Here's how the part is built. I have some questions about the finished solid (model axes, mm). A direction names the side the tool comes from. Round coordinates to 2 decimals unless told otherwise and drop trailing zeros. Loops run counter-clockwise (first coordinate to the right, second up) from the corner with the lowest first, then second, coordinate; pieces in that order, holes last. Notation, with made-up numbers: M -20.75,-40 L -0.75,-40 A13 cw -0.75,-27 Z; hole C 21.25,14 d1. An arc over 180 degrees is marked long. Put each result on its own line as item: value. Start each with the question number.
```python
from build123d import *

# Parameters (mm, degrees)
SKETCH_1_W          = 147
SKETCH_1_H          = 50
SKETCH_1_R          = 1.5
EXTRUDE_1_DEPTH     = 2
CUT_EXTRUDE_1_DEPTH = 2
FILLET_2_DEPTH      = 2
FILLET_3_R          = 4
CUT_EXTRUDE_3_DEPTH = 78.661122835
SKETCH_7_R          = 1.75
CUT_EXTRUDE_4_DEPTH = 78.661122835
CUT_EXTRUDE_5_DEPTH = 10
FILLET_4_R          = 1


with BuildPart() as part:
    # 草图1 → 凸台-拉伸1 (new body)
    with BuildSketch(Plane(origin=(0, 0, 0), x_dir=(1, 0, 0), z_dir=(0, 1, 0))):
        Rectangle(SKETCH_1_W, SKETCH_1_H)
        with Locations(Location((18, -18, 0), (0, 0, 270))):
            Circle(SKETCH_1_R, mode=Mode.SUBTRACT)
        with Locations(Location((-18, -18, 0), (0, 0, 270))):
            Circle(SKETCH_1_R, mode=Mode.SUBTRACT)
        with Locations(Location((-18, 18, 0), (0, 0, 270))):
            Circle(SKETCH_1_R, mode=Mode.SUBTRACT)
        with Locations(Location((18, 18, 0), (0, 0, 270))):
            Circle(SKETCH_1_R, mode=Mode.SUBTRACT)
    extrude(amount=EXTRUDE_1_DEPTH)

    # 草图3 → 切除-拉伸1 (cut)
    with BuildSketch(Plane(origin=(0, 2, 0), x_dir=(1, 0, 0), z_dir=(0, 1, 0))):
        with BuildLine():
            Line((-13.345416088, 16.173843213), (0, 2.828427125))
            Line((0, 2.828427125), (13.345416088, 16.173843213))
            ThreePointArc((13.345416088, 16.173843213), (13.868972045, 20.816843629), (18, 23))
            Line((18, 23), (-18, 23))
            ThreePointArc((-18, 23), (-14.464466094, 21.535533906), (-13, 18))
            ThreePointArc((-13, 18), (-13.087112888, 17.070731352), (-13.345416088, 16.173843213))
        make_face()
        with BuildLine():
            Line((16.173843213, 13.345416088), (2.828427125, 0))
            Line((2.828427125, 0), (16.173843213, -13.345416088))
            ThreePointArc((16.173843213, -13.345416088), (20.816843629, -13.868972045), (23, -18))
            Line((23, -18), (23, 18))
            ThreePointArc((23, 18), (20.816843629, 13.868972045), (16.173843213, 13.345416088))
        make_face()
        with BuildLine():
            Line((0, -2.828427125), (-13.345416088, -16.173843213))
            ThreePointArc((-13.345416088, -16.173843213), (-13.087112888, -17.070731352), (-13, -18))
            ThreePointArc((-13, -18), (-14.464466094, -21.535533906), (-18, -23))
            Line((-18, -23), (18, -23))
            ThreePointArc((18, -23), (13.868972045, -20.816843629), (13.345416088, -16.173843213))
            Line((13.345416088, -16.173843213), (0, -2.828427125))
        make_face()
        with BuildLine():
            ThreePointArc((-23, -18), (-20.816843629, -13.868972045), (-16.173843213, -13.345416088))
            Line((-16.173843213, -13.345416088), (-2.828427125, 0))
            Line((-2.828427125, 0), (-16.173843213, 13.345416088))
            ThreePointArc((-16.173843213, 13.345416088), (-20.816843629, 13.868972045), (-23, 18))
            Line((-23, 18), (-23, -18))
        make_face()
    extrude(amount=-CUT_EXTRUDE_1_DEPTH, mode=Mode.SUBTRACT)

    # 圆角2: read off the stored shape, not the designer's step
    # 圆角2 outline → 圆角2 (add)
    with BuildSketch(Plane(origin=(0, 0, 0), x_dir=(1, 0, 0), z_dir=(0, 1, 0))):
        with BuildLine():
            Line((-23, 18), (-23, 9.05572809))
            ThreePointArc((-23, 9.05572809), (-21.666666667, 12.03715206), (-18.555555556, 13.03096005))
            ThreePointArc((-18.555555556, 13.03096005), (-21.726779962, 14.666666667), (-23, 18))
        make_face()
        with BuildLine():
            ThreePointArc((-18.555555556, -13.03096005), (-21.666666667, -12.03715206), (-23, -9.05572809))
            Line((-23, -9.05572809), (-23, -18))
            ThreePointArc((-23, -18), (-21.726779962, -14.666666667), (-18.555555556, -13.03096005))
        make_face()
        with BuildLine():
            ThreePointArc((13.03096005, -18.555555556), (12.03715206, -21.666666667), (9.05572809, -23))
            Line((9.05572809, -23), (18, -23))
            ThreePointArc((18, -23), (14.666666667, -21.726779962), (13.03096005, -18.555555556))
        make_face()
        with BuildLine():
            ThreePointArc((-9.05572809, -23), (-12.03715206, -21.666666667), (-13.03096005, -18.555555556))
            ThreePointArc((-13.03096005, -18.555555556), (-14.666666667, -21.726779962), (-18, -23))
            Line((-18, -23), (-9.05572809, -23))
        make_face()
        with BuildLine():
            ThreePointArc((18.555555556, 13.03096005), (21.666666667, 12.03715206), (23, 9.05572809))
            Line((23, 9.05572809), (23, 18))
            ThreePointArc((23, 18), (21.726779962, 14.666666667), (18.555555556, 13.03096005))
        make_face()
        with BuildLine():
            ThreePointArc((23, -9.05572809), (21.666666667, -12.03715206), (18.555555556, -13.03096005))
            ThreePointArc((18.555555556, -13.03096005), (21.726779962, -14.666666667), (23, -18))
            Line((23, -18), (23, -9.05572809))
        make_face()
        with BuildLine():
            ThreePointArc((-13.03096005, 18.555555556), (-12.03715206, 21.666666667), (-9.05572809, 23))
            Line((-9.05572809, 23), (-18, 23))
            ThreePointArc((-18, 23), (-14.666666667, 21.726779962), (-13.03096005, 18.555555556))
        make_face()
        with BuildLine():
            ThreePointArc((9.05572809, 23), (12.03715206, 21.666666667), (13.03096005, 18.555555556))
            ThreePointArc((13.03096005, 18.555555556), (14.666666667, 21.726779962), (18, 23))
            Line((18, 23), (9.05572809, 23))
        make_face()
    extrude(amount=FILLET_2_DEPTH)

    # 圆角3
    fillet_3_edges = [part.edges().sort_by_distance(p)[0] for p in [
        (13.345416088, 1, 16.173843213),
        (-13.345416088, 1, 16.173843213),
        (0, 1, 2.828427125),
        (16.173843213, 1, -13.345416088),
        (16.173843213, 1, 13.345416088),
        (2.828427125, 1, 0),
        (-16.173843213, 1, -13.345416088),
        (-2.828427125, 1, 0),
        (-16.173843213, 1, 13.345416088),
        (-13.345416088, 1, -16.173843213),
        (13.345416088, 1, -16.173843213),
        (0, 1, -2.828427125),
    ]]
    fillet(fillet_3_edges, radius=FILLET_3_R)

    # 草图6 → 切除-拉伸3 (cut, through all)
    with BuildSketch(Plane(origin=(0, 2, 0), x_dir=(1, 0, 0), z_dir=(0, 1, 0))):
        Polygon((63.5, -25), (56.57179677, -13), (36.57179677, -13), (29.643593539, -25), align=None)
    cut_extrude_3 = extrude(amount=-CUT_EXTRUDE_3_DEPTH, mode=Mode.SUBTRACT)

    # 镜向1: 切除-拉伸3 across plane
    add(cut_extrude_3.mirror(Plane(origin=(0, 0, 0), x_dir=(0, 0, 1), z_dir=(1, 0, 0))), mode=Mode.SUBTRACT)

    # 草图7 → 切除-拉伸4 (cut, through all)
    with BuildSketch(Plane.XZ):
        with Locations(Location((70.5, 20, 0), (0, 0, 270))):
            Circle(SKETCH_7_R)
        with Locations(Location((70.5, -15, 0), (0, 0, 270))):
            Circle(SKETCH_7_R)
        with Locations(Location((-70.5, -15, 0), (0, 0, 270))):
            Circle(SKETCH_7_R)
        with Locations(Location((-70.5, 20, 0), (0, 0, 270))):
            Circle(SKETCH_7_R)
    extrude(amount=-CUT_EXTRUDE_4_DEPTH, mode=Mode.SUBTRACT)

    # 草图8 → 切除-拉伸5 (cut)
    with BuildSketch(Plane.XZ):
        Polygon((-62.136702063, 8), (-46.57179677, -3.512380307), (-31.006891476, 8), align=None)
        Polygon((-27.643593539, 5.512380307), (-43.208498833, -6), (-27.643593539, -17.512380307), align=None)
        Polygon((-46.57179677, -8.487619693), (-62.136702063, -20), (-31.006891476, -20), align=None)
        Polygon((-65.5, 5.512380307), (-65.5, -17.512380307), (-49.935094706, -6), align=None)
        Polygon((27.643593539, -17.512380307), (43.208498833, -6), (27.643593539, 5.512380307), align=None)
        Polygon((31.006891476, 8), (46.57179677, -3.512380307), (62.136702063, 8), align=None)
        Polygon((49.935094706, -6), (65.5, -17.512380307), (65.5, 5.512380307), align=None)
        Polygon((62.136702063, -20), (46.57179677, -8.487619693), (31.006891476, -20), align=None)
    extrude(amount=-CUT_EXTRUDE_5_DEPTH, mode=Mode.SUBTRACT)

    # 圆角4
    fillet_4_edges = [part.edges().sort_by_distance(p)[0] for p in [
        (27.643593539, 1, -17.512380307),
        (27.643593539, 1, 5.512380307),
        (43.208498833, 1, -6),
        (-65.5, 1, -17.512380307),
        (-65.5, 1, 5.512380307),
        (-49.935094706, 1, -6),
        (-43.208498833, 1, -6),
        (-27.643593539, 1, 5.512380307),
        (-27.643593539, 1, -17.512380307),
        (-62.136702063, 1, -20),
        (-46.57179677, 1, -8.487619693),
        (-31.006891476, 1, -20),
        (62.136702063, 1, -20),
        (31.006891476, 1, -20),
        (46.57179677, 1, -8.487619693),
        (62.136702063, 1, 8),
        (46.57179677, 1, -3.512380307),
        (31.006891476, 1, 8),
        (65.5, 1, -17.512380307),
        (49.935094706, 1, -6),
        (65.5, 1, 5.512380307),
        (-46.57179677, 1, -3.512380307),
        (-62.136702063, 1, 8),
        (-31.006891476, 1, 8),
    ]]
    fillet(fillet_4_edges, radius=FILLET_4_R)


solid = part.part
```
1) If we mould it in two halves opening along X, with no side actions, what happens to faces 1 (the face through (-1, 0, 0)), 2 (the face through (35.77, 0.99, -0.5))? For each: pulls with the +X half, pulls with the -X half, needs draft (parallel to the pull), parting line crosses it, or undercut.
2) On a 3-axis mill with a long thin cutter (end or side, diameter ignored), from which of +Z, -Z, +X, -X, +Y, -Y can I reach the whole of each face in a straight line? I mean faces 3 (the face through (-60.08, 1.01, 19.08)), 4 (the face through (-1, 2, 0)), 5 (the face through (21.63, 0.99, -12.07)). Say none if no direction works.
3) I'm going to push flat-ended pins straight in: P1, Ø5, axis at x = -7, z = 13.5, coming from the +Y side; P2, Ø5.5, axis at x = 70.5, z = 20, coming from the -Y side. Where does each tip first touch, or does it pass through?
4) If I drill on probe 1 along Z at (x, y) = (-70.5, 0.7); probe 2 along Z at (x, y) = (48.5, 1.75); probe 3 along X at (y, z) = (0.65, 20), over which ranges is the centre line in solid material (lowest first)? Write a range as from..to.
5) Suppose I cut it at A-A (x = 70.5). Write out the boundary of the cut face in (y, z).
6) Suppose I cut it at B-B (y = 1.5). State how many separate pieces and enclosed holes the cut face has, plus the area to 3 significant figures.
Results are:
1. face 1: needs draft
1. face 2: undercut
2. face 3: +Z, +Y, -Y
2. face 4: +Z, -Z, +X, -X, +Y
2. face 5: +Y, -Y
3. P1: through
3. P2: y = 0
4. probe 1: -25..-16.75, -13.25..18.25, 21.75..25
4. probe 2: -25..-20, -9.91..-2.09, 8..13
4. probe 3: -73.5..-72.25, -68.75..-60.61, -32.53..-12.93, 12.93..32.53, 60.61..68.75, 72.25..73.5
5. outline: M 0,-25 L 2,-25 L 2,-16.75 L 0,-16.75 Z; M 0,-13.25 L 2,-13.25 L 2,18.25 L 0,18.25 Z; M 0,21.75 L 2,21.75 L 2,25 L 0,25 Z
6. separate pieces: 1
6. enclosed holes: 20
6. area: 3,850 mm²
